Part model, mm, in its own coordinate system. A direction names the side the tool comes from. Coordinates: 2 decimals unless noted, no trailing zeros. Write each loop counter-clockwise with the first axis right and the second up, starting at its lowest first coordinate (ties: lowest second). Pieces come first, ordered by that corner, then holes. Notation, with made-up numbers: (23.25, 60.25) - (81.25, 60.25) arc R27 ccw to (81.25, 84.25) - close; hole circle Ø1 at (-30.75, 54). An arc over 180 degrees is marked (long way). Write each question's results on one line, items separated by ' | '.
from build123d import *

# Parameters (mm, degrees)
SKETCH_1_W      = 33
SKETCH_1_H      = 18.9
SKETCH_1_R      = 2.25
SKETCH_1_R_2    = 0.75
EXTRUDE_1_DEPTH = 2
SKETCH_3_W      = 33.014157098
SKETCH_3_H      = 32
EXTRUDE_2_DEPTH = 2
SKETCH_7_W      = 5.6
SKETCH_7_H      = 16.9
SKETCH_7_R      = 0.75
SKETCH_7_W_2    = 7.6
EXTRUDE_3_DEPTH = 2
SKETCH_8_W      = 33.014157098
SKETCH_8_H      = 18.9
EXTRUDE_4_DEPTH = 2


with BuildPart() as part:
    # 草图1 → 凸台-拉伸1 (new body)
    with BuildSketch(Plane.XY):
        with Locations((0, 9.45)):
            Rectangle(SKETCH_1_W, SKETCH_1_H)
        with Locations((0, 10.9)):
            Circle(SKETCH_1_R, mode=Mode.SUBTRACT)
        with Locations((0, 17.4)):
            Circle(SKETCH_1_R_2, mode=Mode.SUBTRACT)
        with Locations((-6.5, 10.9)):
            Circle(SKETCH_1_R_2, mode=Mode.SUBTRACT)
        with Locations((-12.5, 10.9)):
            Circle(SKETCH_1_R_2, mode=Mode.SUBTRACT)
        with Locations(Location((6.5, 10.9, 0), (0, 0, 180))):
            Circle(SKETCH_1_R_2, mode=Mode.SUBTRACT)
        with Locations(Location((12.5, 10.9, 0), (0, 0, 180))):
            Circle(SKETCH_1_R_2, mode=Mode.SUBTRACT)
    extrude(amount=EXTRUDE_1_DEPTH)

    # 草图3 → 凸台-拉伸2 (add)
    with BuildSketch(Plane.XZ):
        with Locations((0.007078549, 16)):
            Rectangle(SKETCH_3_W, SKETCH_3_H)
    extrude(amount=-EXTRUDE_2_DEPTH)

    # 草图7 → 凸台-拉伸3 (add)
    # profile 1 of 2: a face of its own
    with BuildSketch(Plane(origin=(16.514157098, 0, 0), x_dir=(0, 0, -1), z_dir=(1, 0, 0))):
        with Locations((-29.2, 10.45)):
            Rectangle(SKETCH_7_W, SKETCH_7_H)
        with Locations(Location((-28.1, 10.4, 0), (0, 0, 180))):
            Circle(SKETCH_7_R, mode=Mode.SUBTRACT)
    # profile 2 of 2: a face of its own
    with BuildSketch(Plane(origin=(16.514157098, 0, 0), x_dir=(0, 0, -1), z_dir=(1, 0, 0))):
        with Locations((-5.8, 10.45)):
            Rectangle(SKETCH_7_W_2, SKETCH_7_H)
        with Locations((-7.9, 10.4)):
            Circle(SKETCH_7_R, mode=Mode.SUBTRACT)
    extrude(amount=-EXTRUDE_3_DEPTH)

    # 草图8 → 凸台-拉伸4 (add)
    with BuildSketch(Plane.XY.offset(32)):
        with Locations((0.007078549, 9.45)):
            Rectangle(SKETCH_8_W, SKETCH_8_H)
    extrude(amount=EXTRUDE_4_DEPTH)


solid = part.part
(1) Wall check: line 1 (Y direction, x = 0, z = 1.65); line 2 (Z direction, x = -11, y = 2.75); line 3 (Y direction, x = 15, z = 28). Give the ranges that are in metal, low to high. Write a range as from..to.
Return value:
line 1: y = 0..8.65, 13.15..16.65, 18.15..18.9 | line 2: z = 0..2, 32..34 | line 3: y = 0..9.66, 11.14..18.9
(2) Two-plate mould, pull along Z, no slides. Class faces 1 (the flat face through (0, 7, 0)), 2 (the flat face through (-1, 11, 32)), 3 (the flat face through (0, 2, 17)), 4 (the flat face through (16.514, 1, 17)): released by +Z, released by -Z, zero draft, split by the parting line, or undercut.
Return value:
face 1: released by -Z | face 2: undercut | face 3: undercut | face 4: zero draft
(3) Saw through at A-A on y = 17.4. Count the separate pieces of the cut face and the enclosed holes in it, then the cut area to 3 significant figures.
Return value:
separate pieces: 3 | enclosed holes: 0 | area: 155 mm^2
(4) Saw through at C-C on z = 28.1. Write the cut outline in (x, y).
Return value:
outline: (-16.5, 0) - (16.51, 0) - (16.51, 9.65) - (14.51, 9.65) - (14.51, 2) - (-16.5, 2) - close; (14.51, 11.15) - (16.51, 11.15) - (16.51, 18.9) - (14.51, 18.9) - close
(5) Flat gauge pins, fed straight in: P1, Ø1, axis at x = 11, y = 10, coming from the -Z side; P2, Ø1.7, axis at y = 14.5, z = 28.5, coming from the -X side; P3, Ø1, axis at x = 8, z = 27, coming from the +Y side; P4, Ø1.6, axis at y = 11.5, z = 0.5, coming from the +X side. Where does each tip first touch, or does it go through?
Return value:
P1: stops at z = 0 | P2: stops at x = 14.51 | P3: stops at y = 2 | P4: stops at x = 16.5
(6) 3-axis set-ups, long thin cutter, end or side, ignore diameter. For faces 5 (the flat face through (16, 10, 26.4)), 6 (the cylindrical face through (6.598, 10.156, 0.986)), 7 (the flat face through (2.4, 18.9, 32.4)), 8 (the flat face through (14.514, 11, 6)): which of +Z, -Z, +X, -X, +Y, -Y reach the whole face in a straight line?
Return value:
face 5: +X, -X, +Y | face 6: -Z | face 7: +Z, -Z, +X, -X, +Y | face 8: -X, +Y
(7) Saw through at B-B on x = 12.5. Write the cut outline in (y, z), then the cut area to 3 significant figures.
Return value:
outline: (0, 0) - (10.15, 0) - (10.15, 2) - (2, 2) - (2, 32) - (18.9, 32) - (18.9, 34) - (0, 34) - close; (11.65, 0) - (18.9, 0) - (18.9, 2) - (11.65, 2) - close | area: 133 mm^2
(8) Saw through at D-D on x = 0. Write the cut outline in (y, z).
Return value:
outline: (0, 0) - (8.65, 0) - (8.65, 2) - (2, 2) - (2, 32) - (18.9, 32) - (18.9, 34) - (0, 34) - close; (13.15, 0) - (16.65, 0) - (16.65, 2) - (13.15, 2) - close; (18.15, 0) - (18.9, 0) - (18.9, 2) - (18.15, 2) - close
